from build123d import *

# Parameters (mm, degrees)
F1_DEPTH = 50.8


with BuildPart() as f1:
    # F0 (on Top) → F1 (new body)
    with BuildSketch(Plane.XY):
        with BuildLine():
            Line((-45.975181, 28.836208), (-34.458694, 29.371214))
            ThreePointArc((-34.458694, 29.371214), (-30.05213, 31.032784), (-27.46379, 34.967137))
            Line((-27.46379, 34.967137), (-24.413821, 46.085292))
            ThreePointArc((-24.413821, 46.085292), (-24.632365, 50.789637), (-27.574315, 54.467076))
            Line((-27.574315, 54.467076), (-37.205817, 60.803468))
            ThreePointArc((-37.205817, 60.803468), (-41.747449, 62.049343), (-46.154014, 60.387773))
            Line((-46.154014, 60.387773), (-55.156579, 53.185723))
            ThreePointArc((-55.156579, 53.185723), (-57.744918, 49.251371), (-57.526374, 44.547026))
            Line((-57.526374, 44.547026), (-53.458763, 33.759522))
            ThreePointArc((-53.458763, 33.759522), (-50.516813, 30.082084), (-45.975181, 28.836208))
        make_face()
    extrude(amount=F1_DEPTH)


solid = f1.part
For this review, take the finished solid that the model builds, in its own axes (mm). Give positions to 0.01 mm unless a question says otherwise; leave off trailing zeros. Order: outer loops, then holes, each group sorted by start corner. A loop starts at its lowest first (then second) coordinate and runs counter-clockwise, first axis right, second up. Notation, with made-up numbers: M 6.25,85 L 34.25,85 A6 ccw 34.25,93 Z; hole C -36.5,-38.5 d3. An arc over 180 degrees is marked long. Answer in a Markdown table with one row per item. Add a question column.
(1) Consider section C-C on x = -39.5. State the section outline as (y, z) points, and give its area (3 significant figures).
(2) Consider section B-B on y = 39.5. State the section outline as (x, z) points.
(3) Wall thickness on probe 1 along Y at (x, z) = (-30, 49.5); probe 2 along X at (y, z) = (46, 43); probe 3 along X at (y, z) = (37, 39): over which ranges is each line inside the solid? List them lowest first. Write a range as [from, to].
(4) Consider section A-A on z = 6.5. State the section outline as (x, y) points, and give its area (3 significant figures).
(5) For pin 1 (6 mm diameter, centred on y = 48.5, z = 17, fed in from -X); pin 2 (1.5 mm diameter, centred on x = -47, z = 24.5, fed in from +Y); pin 3 (6 mm diameter, centred on x = -53, z = 13.5, fed in from -Y); pin 4 (12 mm diameter, centred on x = -33, z = 24, fed in from -Y), all flat-tipped, find the tip position at first contact; note any pin that passes through.
Evaluation:
| question | item | result |
|---|---|---|
| 1 | outline | M 29.14,0 L 61.82,0 L 61.82,50.8 L 29.14,50.8 Z |
| 1 | area | 1,660 mm^2 |
| 2 | outline | M -55.62,0 L -26.22,0 L -26.22,50.8 L -55.62,50.8 Z |
| 3 | probe 1 | y = [31.07, 56.06] |
| 3 | probe 2 | x = [-57.92, -24.44] |
| 3 | probe 3 | x = [-54.68, -26.91] |
| 4 | outline | M -57.53,44.55 L -53.46,33.76 A7.62 ccw -45.98,28.84 L -34.46,29.37 A7.62 ccw -27.46,34.97 L -24.41,46.09 A7.62 ccw -27.57,54.47 L -37.21,60.8 A7.62 ccw -46.15,60.39 L -55.16,53.19 A7.62 ccw Z |
| 4 | area | 850 mm^2 |
| 5 | pin 1 | stops at x = -58.02 |
| 5 | pin 2 | stops at y = 60.31 |
| 5 | pin 3 | stops at y = 29.77 |
| 5 | pin 4 | stops at y = 29.16 |
